from build123d import *

# Parameters (mm, degrees)
SKETCH1_W            = 40.5
SKETCH1_H            = 20
BOSS_EXTRUDE1_DEPTH  = 36.1
BOSS_EXTRUDE2_DEPTH  = 2.5
BOSS_EXTRUDE3_DEPTH  = 1
FILLET1_R            = 1
FILLET1_OF_MIRROR1_R = 1
CHAMFER1_SIZE        = 3
CHAMFER1_SIZE2       = 15
SKETCH4_R            = 2.5
BOSS_EXTRUDE4_DEPTH  = 6
SKETCH5_R            = 10.5
BOSS_EXTRUDE5_DEPTH  = 2


with BuildPart() as part:
    # Sketch1 → Boss-Extrude1 (new body)
    with BuildSketch(Plane.XY):
        Rectangle(SKETCH1_W, SKETCH1_H)
    extrude(amount=BOSS_EXTRUDE1_DEPTH)

    # Sketch2 → Boss-Extrude2 (add)
    with BuildSketch(Plane(origin=(0, 0, 26.1), x_dir=(-1, 0, 0), z_dir=(0, 0, -1))):
        with BuildLine():
            Line((-20.25, 9), (-27.75, 9))
            Line((-27.75, 9), (-27.75, 6))
            Line((-27.75, 6), (-27.265564437, 6))
            ThreePointArc((-27.265564437, 6), (-23, 5), (-27.265564437, 4))
            Line((-27.265564437, 4), (-27.75, 4))
            Line((-27.75, 4), (-27.75, -4))
            Line((-27.75, -4), (-27.265564437, -4))
            ThreePointArc((-27.265564437, -4), (-23, -5), (-27.265564437, -6))
            Line((-27.265564437, -6), (-27.75, -6))
            Line((-27.75, -6), (-27.75, -9))
            Line((-27.75, -9), (-20.25, -9))
            Line((-20.25, -9), (-20.25, 9))
        make_face()
    boss_extrude2 = extrude(amount=-BOSS_EXTRUDE2_DEPTH)

    # Sketch3 → Boss-Extrude3 (add)
    with BuildSketch(Plane.XY.offset(28.6)):
        with BuildLine():
            Line((20.25, 1), (23.25, 1))
            ThreePointArc((23.25, 1), (24.25, 0), (23.25, -1))
            Line((23.25, -1), (20.25, -1))
            Line((20.25, -1), (20.25, 1))
        make_face()
    boss_extrude3 = extrude(amount=BOSS_EXTRUDE3_DEPTH)

    # Fillet1
    fillet1_edges = [part.edges().sort_by_distance(p)[0] for p in [
        (27.75, -9, 27.35),
        (27.75, 9, 27.35),
    ]]
    fillet(fillet1_edges, radius=FILLET1_R)

    # Mirror1: Boss-Extrude2, Boss-Extrude3 across plane
    add(boss_extrude2.mirror(Plane(origin=(0, 0, 0), x_dir=(0, 0, 1), z_dir=(1, 0, 0))))
    add(boss_extrude3.mirror(Plane(origin=(0, 0, 0), x_dir=(0, 0, 1), z_dir=(1, 0, 0))))

    # Fillet1 of Mirror1
    fillet1_of_mirror1_edges = [part.edges().sort_by_distance(p)[0] for p in [
        (-27.75, -9, 27.35),
        (-27.75, 9, 27.35),
    ]]
    fillet(fillet1_of_mirror1_edges, radius=FILLET1_OF_MIRROR1_R)

    # Chamfer1
    chamfer1_edges = [part.edges().sort_by_distance(p)[0] for p in [
        (-20.25, 0, 36.1),
    ]]
    chamfer1_side = [part.faces().sort_by_distance(p)[0] for p in [
        (-20.25, 0, 17.397259259),
    ]]
    chamfer(chamfer1_edges, length=CHAMFER1_SIZE, length2=CHAMFER1_SIZE2, reference=chamfer1_side[0])

    # Sketch4 → Boss-Extrude4 (add)
    with BuildSketch(Plane.XY.offset(36.1)):
        with Locations((9.85, 0)):
            Circle(SKETCH4_R)
    extrude(amount=BOSS_EXTRUDE4_DEPTH)

    # Sketch5 → Boss-Extrude5 (add)
    with BuildSketch(Plane.XY.offset(42.1)):
        with Locations((9.85, 0)):
            Circle(SKETCH5_R)
    extrude(amount=BOSS_EXTRUDE5_DEPTH)


solid = part.part
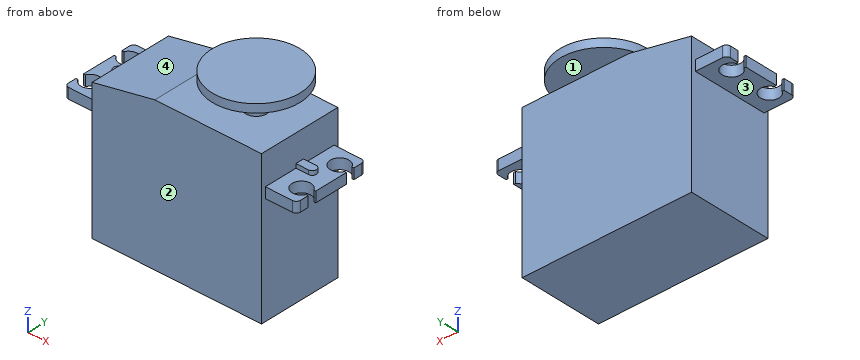
Check sheet for the modelled part. Datum: model origin and axes. Units: mm. Face numbers are marked on the shaded views. Round coordinates to 2 decimals unless told otherwise and drop trailing zeros. Loops run counter-clockwise (first coordinate to the right, second up) from the corner with the lowest first, then second, coordinate; pieces in that order, holes last. Notation, with made-up numbers: (36, 12) -> (57, 12) arc R6 cw to (57, 22) -> close; hole circle Ø7 at (-26.5, 16.25). An arc over 180 degrees is marked (long way). Put each result on its own line as item: value. Start each with the question number.
1. Section check C-C (x = 2). Enter the section's corners in (y, z), plus the area to 3 significant figures.
2. Section check A-A (x = 25.25). Enter the section's corners in (y, z), plus the area to 3 significant figures.
3. Draft check along Z on the marked faces 1, 2, 3 and 4. Enter one of: +Z half, -Z half, draft (parallel to the pull), parting line (faces both ways), or undercut.
4. Section check D-D (y = 0). Enter the section's corners in (x, z), plus the area to 3 significant figures.
5. Section check B-B (y = 5). Enter the section's corners in (x, z).
6. Scan lines: probe 1 along Y at (x, z) = (25, 27); probe 2 along Z at (x, y) = (7, 5); probe 3 along X at (y, z) = (2.5, 25). Record each from-to range of solid material in increasing order.
7. Gauge pin test, flat ends, axial feed: pin 1 (18 mm diameter, centred on x = -8.5, z = 20.5, fed in from -Y); pin 2 (6 mm diameter, centred on y = -1.5, z = 39, fed in from +X); pin 3 (3 mm diameter, centred on x = -3.5, z = 25.5, fed in from +Y); pin 4 (10 mm diameter, centred on x = 11, z = 38, fed in from -Y). Record the tip position at first contact, or that the pin passes through.
Findings:
1. outline: (-10, 0) -> (10, 0) -> (10, 36.1) -> (-10, 36.1) -> close; (-6.97, 42.1) -> (6.97, 42.1) -> (6.97, 44.1) -> (-6.97, 44.1) -> close
1. area: 750 mm^2
2. outline: (-9, 26.1) -> (-7.25, 26.1) -> (-7.25, 28.6) -> (-9, 28.6) -> close; (-2.75, 26.1) -> (2.75, 26.1) -> (2.75, 28.6) -> (-2.75, 28.6) -> close; (7.25, 26.1) -> (9, 26.1) -> (9, 28.6) -> (7.25, 28.6) -> close
2. area: 22.5 mm^2
3. face 1: undercut
3. face 2: draft
3. face 3: -Z half
3. face 4: +Z half
4. outline: (-27.75, 26.1) -> (-20.25, 26.1) -> (-20.25, 0) -> (20.25, 0) -> (20.25, 26.1) -> (27.75, 26.1) -> (27.75, 28.6) -> (24.25, 28.6) -> (24.25, 29.6) -> (20.25, 29.6) -> (20.25, 36.1) -> (12.35, 36.1) -> (12.35, 42.1) -> (20.35, 42.1) -> (20.35, 44.1) -> (-0.65, 44.1) -> (-0.65, 42.1) -> (7.35, 42.1) -> (7.35, 36.1) -> (-5.25, 36.1) -> (-20.25, 33.1) -> (-20.25, 29.6) -> (-24.25, 29.6) -> (-24.25, 28.6) -> (-27.75, 28.6) -> close
4. area: 1,560 mm^2
5. outline: (-23, 26.1) -> (-20.25, 26.1) -> (-20.25, 0) -> (20.25, 0) -> (20.25, 26.1) -> (23, 26.1) -> (23, 28.6) -> (20.25, 28.6) -> (20.25, 36.1) -> (-5.25, 36.1) -> (-20.25, 33.1) -> (-20.25, 28.6) -> (-23, 28.6) -> close; (0.62, 42.1) -> (19.08, 42.1) -> (19.08, 44.1) -> (0.62, 44.1) -> close
6. probe 1: y = -9 to -7.24, -2.76 to 2.76, 7.24 to 9
6. probe 2: z = 0 to 36.1, 42.1 to 44.1
6. probe 3: x = -20.25 to 20.25
7. pin 1: stops at y = -10
7. pin 2: stops at x = 20.25
7. pin 3: stops at y = 10
7. pin 4: stops at y = -10.5
